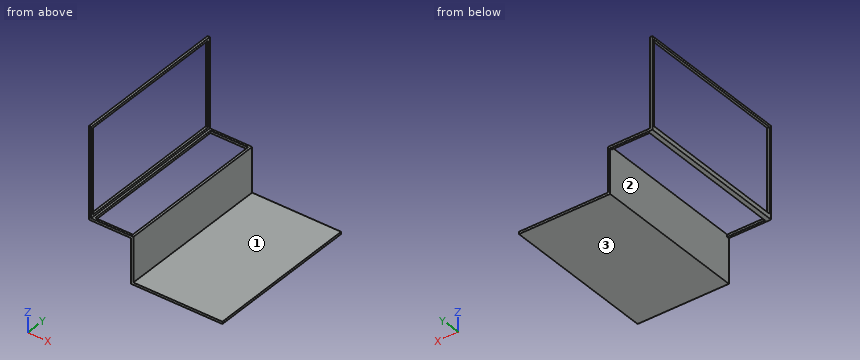
```python
from build123d import *

# Parameters (mm, degrees)
F0_W     = 25.4
F0_H     = 25.4
F0_H_2   = 1000
F1_DEPTH = 1750
F2_W     = 423.8
F2_H     = 1699.2
F3_DEPTH = 25.4
F4_W     = 1699.2
F4_H     = 949.2
F5_DEPTH = 25.4


with BuildPart() as f1:
    # F0 (on Front) → F1 (new body)
    with BuildSketch(Plane.XZ):
        Polygon((1000, 0), (0, 0), (0, 500), (-474.6, 500), (-474.6, 474.6), (-25.4, 474.6), (-25.4, -25.4), (1000, -25.4), align=None)
        with Locations((-487.3, 487.3)):
            Rectangle(F0_W, F0_H)
        with Locations((-487.3, 1000)):
            Rectangle(F0_W, F0_H_2)
    extrude(amount=F1_DEPTH)

    # F2 (on face) → F3 (cut)
    with BuildSketch(Plane.XY.offset(500)):
        with Locations((-237.3, -875)):
            Rectangle(F2_W, F2_H)
    extrude(amount=-F3_DEPTH, mode=Mode.SUBTRACT)

    # F4 (on face) → F5 (cut)
    with BuildSketch(Plane.YZ.offset(-474.6)):
        with Locations((-875, 1000)):
            Rectangle(F4_W, F4_H)
    extrude(amount=-F5_DEPTH, mode=Mode.SUBTRACT)


solid = f1.part
```
The listing builds one solid part. Answer for the finished solid, in the listing's coordinates (mm). Face numbers are marked on the shaded views. Round coordinates to 2 decimals unless told otherwise and drop trailing zeros. Write each loop counter-clockwise with the first axis right and the second up, starting at its lowest first coordinate (ties: lowest second). Pieces come first, ordered by that corner, then holes. Notation, with made-up numbers: (37, 3.5) -> (60, 3.5) arc R6 cw to (60, 14.5) -> close; hole circle Ø5 at (83, 18). An arc over 180 degrees is marked (long way). Answer as a JSON object with one key per item and string values. Group by question number.
Q1. Each of these flat-tipped pins is pushed along its axis until it touches: pin 1 Ø20.5 at (y, z) = (-685, 493.5) entering from +X; pin 2 Ø3 at (y, z) = (-1405.5, 204) entering from -X. Where does it stop, or does it pass through?
Q2. Straight lines are drawn through the part: line 1 along X through (y, z) = (-215, 483.5); line 2 along Z through (x, y) = (548, -630.5). For each, find the intervals that lie inside material, in ascending order.
Q3. Section C-C (x = 526.5) is taken. Write down the section's boundary in (y, z), plus the area to 4 significant figures.
Q4. Section B-B (z = 751) is taken. Write down the section's boundary in (x, y).
Q5. Determine the mould class of the marked faces 1, 2 and 3 for opening direction Z: pulls with the +Z half, pulls with the -Z half, needs draft (parallel to the pull), parting line crosses it, or undercut.
Q6. Section A-A (y = -1343) is taken. Write down the section's boundary in (x, z), plus the area to 3 significant figures.
Check values:
{
 "1": {"pin 1": "x = 0", "pin 2": "x = -25.4"},
 "2": {"line 1": "-500 to -449.2, -25.4 to 0", "line 2": "-25.4 to 0"},
 "3": {"outline": "(-1750, -25.4) -> (0, -25.4) -> (0, 0) -> (-1750, 0) -> close", "area": "44,450 mm^2"},
 "4": {"outline": "(-500, -1750) -> (-474.6, -1750) -> (-474.6, -1724.6) -> (-500, -1724.6) -> close; (-500, -25.4) -> (-474.6, -25.4) -> (-474.6, 0) -> (-500, 0) -> close"},
 "5": {"face 1": "pulls with the +Z half", "face 2": "needs draft", "face 3": "pulls with the -Z half"},
 "6": {"outline": "(-500, 474.6) -> (-449.2, 474.6) -> (-449.2, 500) -> (-474.6, 500) -> (-474.6, 525.4) -> (-500, 525.4) -> close; (-500, 1474.6) -> (-474.6, 1474.6) -> (-474.6, 1500) -> (-500, 1500) -> close; (-25.4, -25.4) -> (1000, -25.4) -> (1000, 0) -> (0, 0) -> (0, 500) -> (-25.4, 500) -> close", "area": "41,300 mm^2"}
}
